Geometry: final body of the model. Coordinates: model frame, mm. A direction names the side the tool comes from. Coordinates: 2 decimals unless noted, no trailing zeros. One line per item, written item: value.
```python
from build123d import *

# Parameters (mm, degrees)
F1_DEPTH = 250.825
F2_R     = 2.54
F3_R     = 2.54
F4_R     = 2.54
F6_W     = 6.35
F6_H     = 501.65
F7_DEPTH = 7.62
F8_DEPTH = 17.4635001


# Not quite as in the source:
# - ends of sketch curves that miss each other by under 0.0002 mm in the source are joined


with BuildPart() as f1:
    # F0 (on Top) → F1 (new body, symmetric)
    with BuildSketch(Plane.XY):
        with BuildLine():
            Line((15.875, 5.55625), (15.875, 8.73125))
            Line((15.875, 8.73125), (-15.875, 8.73125))
            Line((-15.875, 8.73125), (-15.875, -0.79375))
            Line((-15.875, -0.79375), (-12.7, -0.79375))
            ThreePointArc((-12.7, -0.79375), (-9.8710707302, -6.4481459867), (-3.9751, -8.73125))
            Line((-3.9751, -8.73125), (-3.96875, -8.73125))
            ThreePointArc((-3.96875, -8.73125), (1.9312218072, -6.4502821485), (4.7625, -0.79375))
            Line((4.7625, -0.79375), (7.9375, -0.79375))
            ThreePointArc((7.9375, -0.79375), (10.9883747468, 3.5285940665), (15.875, 5.55625))
        make_face()
    extrude(amount=F1_DEPTH, both=True)

    # F2
    f2_edges = [f1.edges().sort_by_distance(p)[0] for p in [
        (7.9375, -0.79375, 0),
    ]]
    fillet(f2_edges, radius=F2_R)

    # F3
    f3_edges = [f1.edges().sort_by_distance(p)[0] for p in [
        (-12.7, -0.79375, 0),
    ]]
    fillet(f3_edges, radius=F3_R)

    # F4
    f4_edges = [f1.edges().sort_by_distance(p)[0] for p in [
        (4.7625, -0.79375, 0),
    ]]
    fillet(f4_edges, radius=F4_R)

    # F6 (on face) → F7 (cut)
    with BuildSketch(Plane(origin=(0, 8.73125, 0), x_dir=(-1, 0, 0), z_dir=(0, 1, 0))):
        with Locations((12.7, 0)):
            Rectangle(F6_W, F6_H)
    extrude(amount=-F7_DEPTH, mode=Mode.SUBTRACT)

    # F5 (on face) → F8 (cut, through all)
    with BuildSketch(Plane(origin=(0, 8.73125, 0), x_dir=(-1, 0, 0), z_dir=(0, 1, 0))):
        Polygon((15.875, -250.825), (15.875, -219.075), (-15.875, -250.825), align=None)
        Polygon((-15.875, 250.825), (15.875, 219.075), (15.875, 250.825), align=None)
    extrude(amount=-F8_DEPTH, mode=Mode.SUBTRACT)


solid = f1.part
```
(1) First-contact query: pin 1 (4 mm diameter, centred on y = 5.5, z = -10.5, fed in from -X) (3 decimals); pin 2 (1 mm diameter, centred on x = -12, y = -3.5, fed in from +Z); pin 3 (1 mm diameter, centred on x = -8, z = -180.5, fed in from -Y); pin 4 (2 mm diameter, centred on x = 6.5, y = -2, fed in from -Z). Flat tips, straight axial feed; report the tip coordinate or a pass-through.
Responses:
pin 1: stops at x = -9.525
pin 2: stops at z = 223.45
pin 3: stops at y = -7.99
pin 4: passes through
(2) Reachability of faces 1 (the flat face through (-9.525, 5, -3)), 2 (the cylindrical face through (1.17, -7.07, 3.35)) from +Z, -Z, +X, -X, +Y, -Y: full face, straight path, thin tool, end or side. Return the list, or none.
Responses:
face 1: +Z, -Z, -X, +Y
face 2: +Z, -Z, +X, -Y
(3) Line query: line 1 (Y direction, x = -5, z = 168); line 2 (X direction, y = 0.5, z = 28) (3 decimals); line 3 (X direction, y = 1, z = 27) (3 decimals). Output: solid intervals per line, ascending. Write a range as [from, to].
Responses:
line 1: y = [-8.67, 8.73]
line 2: x = [-15.875, 8.494]
line 3: x = [-15.875, 8.776]
